CAD build for the part. Positions are in the model's coordinates, mm. Face numbers are marked on the shaded views. A direction names the side the tool comes from. Round coordinates to 2 decimals unless told otherwise and drop trailing zeros. Answer as CSV lines item,"result". Start each with the question number.
```python
from build123d import *

# Parameters (mm, degrees)
SKETCH2_R           = 57.15
BOSS_EXTRUDE1_DEPTH = 8.35
CUT_EXTRUDE1_REACH  = 10.35
SKETCH6_R           = 3.175
SKETCH7_R           = 14.732
SKETCH7_R_2         = 1.778
CUT_EXTRUDE2_DEPTH  = 9.35
SKETCH8_R           = 5.042
CUT_EXTRUDE3_DEPTH  = 9.35
CIRPATTERN1_COUNT   = 6
CHAMFER1_SIZE       = 1


with BuildPart() as part:
    # Sketch2 → Boss-Extrude1 (new body)
    with BuildSketch(Plane(origin=(0, 0, 0), x_dir=(1, 0, 0), z_dir=(0, 1, 0))):
        Circle(SKETCH2_R)
    extrude(amount=BOSS_EXTRUDE1_DEPTH)

    # Sketch6 → Cut-Extrude1 (cut, up to next)
    with BuildSketch(Plane(origin=(0, 8.35, 0), x_dir=(1, 0, 0), z_dir=(0, 1, 0)), mode=Mode.PRIVATE) as cut_extrude1_sk1:
        with Locations((-26.1629, -26.1629)):
            Circle(SKETCH6_R)
    cut_extrude1_tool1 = extrude(cut_extrude1_sk1.sketch, amount=-CUT_EXTRUDE1_REACH, mode=Mode.PRIVATE) & part.part
    add(cut_extrude1_tool1.solids().sort_by_distance((-26.1629, 8.35, 26.1629))[0], mode=Mode.SUBTRACT)
    # Sketch6 → Cut-Extrude1 (cut, up to next)
    with BuildSketch(Plane(origin=(0, 8.35, 0), x_dir=(1, 0, 0), z_dir=(0, 1, 0)), mode=Mode.PRIVATE) as cut_extrude1_sk2:
        with Locations((26.1629, -26.1629)):
            Circle(SKETCH6_R)
    cut_extrude1_tool2 = extrude(cut_extrude1_sk2.sketch, amount=-CUT_EXTRUDE1_REACH, mode=Mode.PRIVATE) & part.part
    add(cut_extrude1_tool2.solids().sort_by_distance((26.1629, 8.35, 26.1629))[0], mode=Mode.SUBTRACT)
    # Sketch6 → Cut-Extrude1 (cut, up to next)
    with BuildSketch(Plane(origin=(0, 8.35, 0), x_dir=(1, 0, 0), z_dir=(0, 1, 0)), mode=Mode.PRIVATE) as cut_extrude1_sk3:
        with Locations((-26.1629, 26.163103615)):
            Circle(SKETCH6_R)
    cut_extrude1_tool3 = extrude(cut_extrude1_sk3.sketch, amount=-CUT_EXTRUDE1_REACH, mode=Mode.PRIVATE) & part.part
    add(cut_extrude1_tool3.solids().sort_by_distance((-26.1629, 8.35, -26.163104))[0], mode=Mode.SUBTRACT)
    # Sketch6 → Cut-Extrude1 (cut, up to next)
    with BuildSketch(Plane(origin=(0, 8.35, 0), x_dir=(1, 0, 0), z_dir=(0, 1, 0)), mode=Mode.PRIVATE) as cut_extrude1_sk4:
        with Locations((26.1629, 26.163103615)):
            Circle(SKETCH6_R)
    cut_extrude1_tool4 = extrude(cut_extrude1_sk4.sketch, amount=-CUT_EXTRUDE1_REACH, mode=Mode.PRIVATE) & part.part
    add(cut_extrude1_tool4.solids().sort_by_distance((26.1629, 8.35, -26.163104))[0], mode=Mode.SUBTRACT)

    # Sketch7 → Cut-Extrude2 (cut, through all)
    with BuildSketch(Plane(origin=(0, 8.35, 0), x_dir=(1, 0, 0), z_dir=(0, 1, 0))):
        with Locations((30, 0.269903496)):
            Circle(SKETCH7_R)
        with Locations((16.54, -13.194096504)):
            Circle(SKETCH7_R_2)
        with Locations((16.54, 13.729903496)):
            Circle(SKETCH7_R_2)
        with Locations((43.46, 13.729903496)):
            Circle(SKETCH7_R_2)
        with Locations((43.46, -13.194096504)):
            Circle(SKETCH7_R_2)
    extrude(amount=-CUT_EXTRUDE2_DEPTH, mode=Mode.SUBTRACT)

    # Sketch8 → Cut-Extrude3 (cut, through all)
    with BuildSketch(Plane(origin=(0, 8.35, 0), x_dir=(1, 0, 0), z_dir=(0, 1, 0))):
        Circle(SKETCH8_R)
        with BuildLine():
            Line((4.098780306, 34.063103615), (-4.098780306, 34.063103615))
            ThreePointArc((-4.098780306, 34.063103615), (0, 17.263103615), (4.098780306, 34.063103615))
        make_face()
        with BuildLine():
            Line((4.098780306, -34.0629), (-4.098780306, -34.0629))
            ThreePointArc((-4.098780306, -34.0629), (0, -17.2629), (4.098780306, -34.0629))
        make_face()
        with BuildLine():
            Line((-36.1129, 5.249761899), (-36.1129, -5.249761899))
            ThreePointArc((-36.1129, -5.249761899), (-14.9129, 0), (-36.1129, 5.249761899))
        make_face()
    extrude(amount=-CUT_EXTRUDE3_DEPTH, mode=Mode.SUBTRACT)

    # Sketch16 → #6-32 Tapped Hole1 (revolve, cut)
    with BuildSketch(Plane(origin=(0, 4.175, -57.15), x_dir=(0, 1, 0), z_dir=(1, 0, 0))):
        Polygon((0, 0), (0, 13.81269403), (1.35255, 13), (1.35255, 0), align=None)
    f_6_32_tapped_hole1 = revolve(axis=Axis((0, 4.175, -63.5), (0, 0, 1)), mode=Mode.SUBTRACT)

    # CirPattern1: #6-32 Tapped Hole1 ×6 about axis
    cirpattern1_axis = Axis((0, 0, 0), (0, 1, 0))
    for i in range(1, CIRPATTERN1_COUNT):
        add(f_6_32_tapped_hole1.rotate(cirpattern1_axis, i * 360 / CIRPATTERN1_COUNT), mode=Mode.SUBTRACT)

    # Chamfer1
    chamfer1_edges = [part.edges().sort_by_distance(p)[0] for p in [
        (-57.15, 0, 0),
        (-57.15, 8.35, 0),
    ]]
    chamfer(chamfer1_edges, length=CHAMFER1_SIZE)


solid = part.part
```
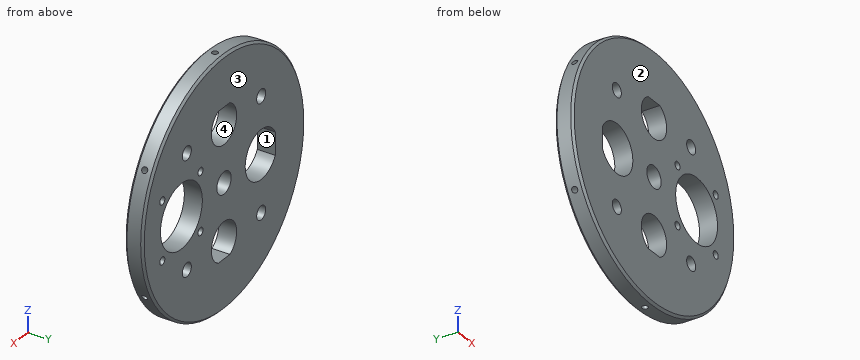
Q1. Drop flat-ended pins along their axis: P1, Ø4, axis at y = 3.5, z = 27, coming from the +X side; P2, Ø1.5, axis at y = 2.5, z = 39.5, coming from the +X side; P3, Ø1, axis at x = -43.5, y = 5.5, coming from the -Z side. Give the stop position or say it passes through.
Q2. Probe line 1 along Z through (x, y) = (4.5, 6.25); line 2 along X through (y, z) = (3.75, 27.5); line 3 along Z through (x, y) = (1.5, 3). List the from-to ranges inside material, lowest first. Write a range as from..to.
Q3. Mould opens along Z. For the marked faces 3 and 4 say: +Z half, -Z half, draft (parallel to the pull), parting line (faces both ways), or undercut.
Q4. Tool access for the marked faces 1 and 2: list every direction of +Z, -Z, +X, -X, +Y, -Y with a clear straight run to the whole face (end or side of a thin tool).
Answer:
1,P1,"stops at x = 51.39"
1,P2,"stops at x = 42.01"
1,P3,"stops at z = -37.64"
2,line 1,"z = -56.97..-33.84, -18.48..-2.27, 2.27..18.48, 33.84..56.97"
2,line 2,"x = -45.06..-29.04, -23.28..-8.8, 8.8..23.28, 29.04..45.06"
2,line 3,"z = -57.13..-34.06, -17.39..-4.81, 4.81..17.39, 34.06..57.13"
3,face 3,"draft"
3,face 4,"undercut"
4,face 1,"+Y, -Y"
4,face 2,"+Z, -Z, +X, -X, -Y"
